Design review of the part shown in the three views and the two pictorial views. Dimensions are in mm from the part's minimum x, y and z. A direction names the side the tool comes from. Give positions to 0.01 mm unless a question says otherwise; leave off trailing zeros. Order: outer loops, then holes, each group sorted by start corner. A loop starts at its lowest first (then second) coordinate and runs counter-clockwise, first axis right, second up.
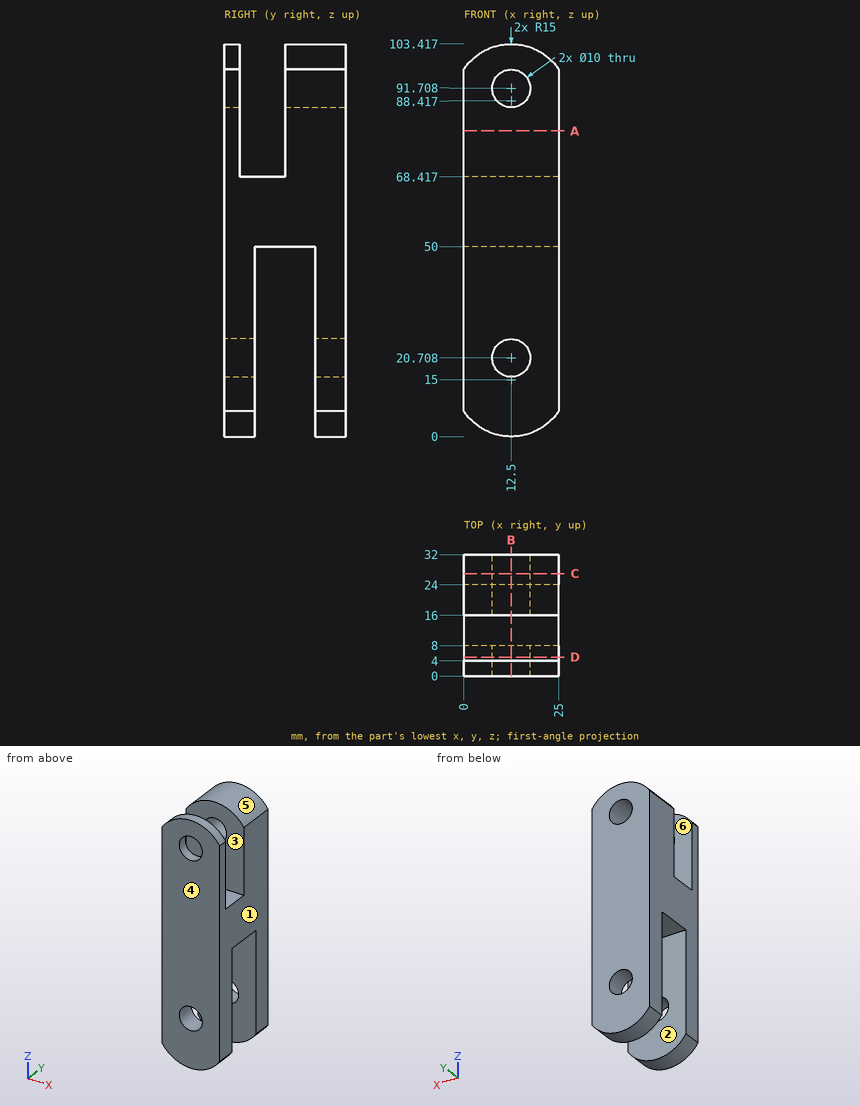
1) We need section D-D on y = 5. Give the boundary of the cut face in (x, z).
Answer sheet:
outline: (0, 6.71) arc R15 ccw to (25, 6.71) - (25, 68.42) - (0, 68.42) - close; hole circle Ø10 at (12.5, 20.71)
2) We need section A-A on z = 80.5. Give the boundary of the cut face in (x, y).
Answer sheet:
outline: (0, 0) - (25, 0) - (25, 4) - (0, 4) - close; (0, 16) - (25, 16) - (25, 32) - (0, 32) - close
3) Clearance check with flat-ended pins moving along their axes: pin 1 (4 mm diameter, centred on x = 9.5, y = 11.5, fed in from +Z); pin 2 (6 mm diameter, centred on x = 19, y = 4, fed in from -Z); pin 3 (8 mm diameter, centred on x = 12, y = 18, fed in from -Z). State where each tip first meets the part, or that it passes through.
Answer sheet:
pin 1: stops at z = 68.42
pin 2: stops at z = 0.41
pin 3: stops at z = 50
4) Tool access review of the marked faces 1, 2 and 3: name each direction out of +Z, -Z, +X, -X, +Y, -Y from which nothing blocks a thin tool from reaching the whole face with its end or side.
Answer sheet:
face 1: +Z, -Z, +X, +Y, -Y
face 2: -Z, +X, -X
face 3: +Z, +X, -X
5) We need section B-B on x = 12.5. Give the boundary of the cut face in (y, z), then the cut area to 3 significant figures.
Answer sheet:
outline: (0, 0) - (8, 0) - (8, 15.71) - (0, 15.71) - close; (0, 25.71) - (8, 25.71) - (8, 50) - (24, 50) - (24, 25.71) - (32, 25.71) - (32, 86.71) - (16, 86.71) - (16, 68.42) - (4, 68.42) - (4, 86.71) - (0, 86.71) - close; (0, 96.71) - (4, 96.71) - (4, 103.42) - (0, 103.42) - close; (16, 96.71) - (32, 96.71) - (32, 103.42) - (16, 103.42) - close; (24, 0) - (32, 0) - (32, 15.71) - (24, 15.71) - close
area: 1,730 mm2
6) We need section C-C on y = 27. Give the boundary of the cut face in (x, z).
Answer sheet:
outline: (0, 6.71) arc R15 ccw to (25, 6.71) - (25, 96.71) arc R15 ccw to (0, 96.71) - close; hole circle Ø10 at (12.5, 20.71); hole circle Ø10 at (12.5, 91.71)
7) To check wall thickness, follow line 1 (Y direction, x = 21, z = 38); line 2 (Y direction, x = 21.5, z = 69.5); line 3 (Z direction, x = 21.5, y = 14.5). State the ranges of each line that lie inside material, in increasing order.
Answer sheet:
line 1: y = 0 to 8, 24 to 32
line 2: y = 0 to 4, 16 to 32
line 3: z = 50 to 68.42
8) Draft analysis for pull direction Y (two halves, no side actions). For the marked faces 4, 5 and 6, state which applies: +Y half, -Y half, draft (parallel to the pull), parting line (faces both ways), or undercut.
Answer sheet:
face 4: -Y half
face 5: draft
face 6: undercut
